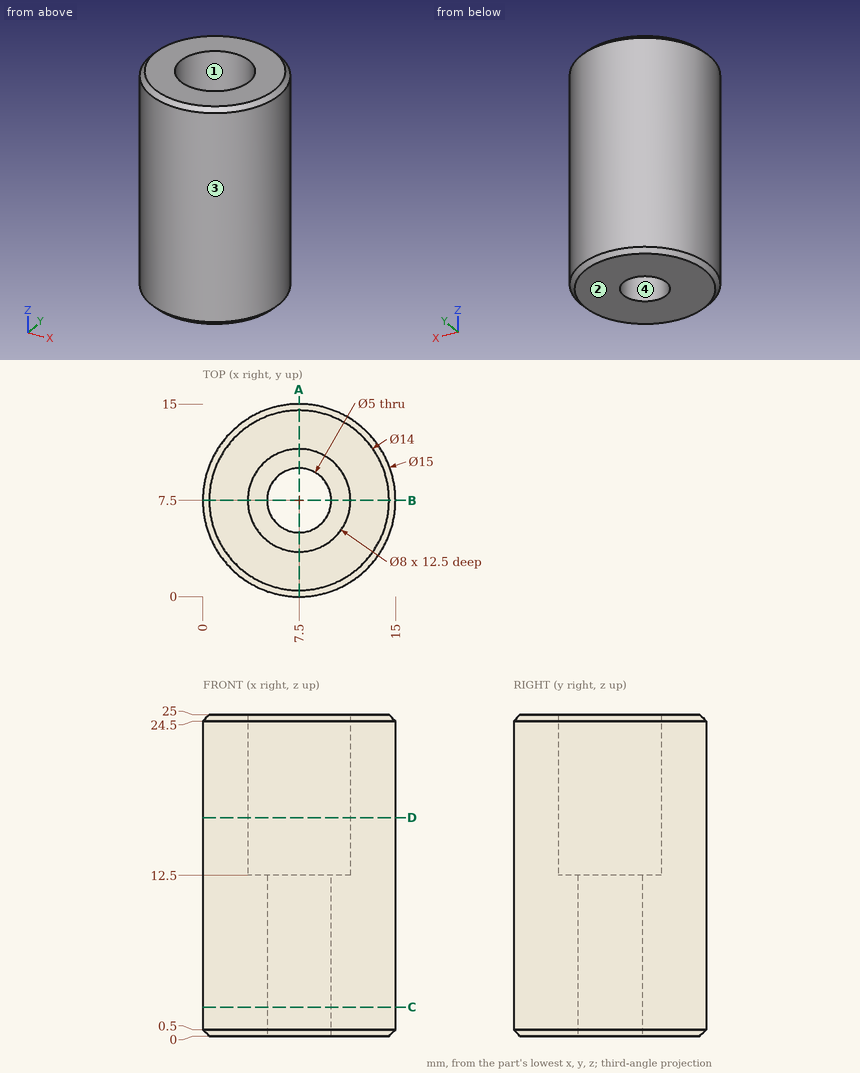
Geometry check sheet. Reference: drawing and pictorial views, mm from the part's lowest x, y, z. Round coordinates to 2 decimals unless told otherwise and drop trailing zeros. Loops run counter-clockwise (first coordinate to the right, second up) from the corner with the lowest first, then second, coordinate; pieces in that order, holes last. Notation, with made-up numbers: M 33.25,32 L 55.25,32 A34 ccw 55.25,69 Z; hole C 2.25,20 d7. An arc over 180 degrees is marked long. One line per item, written item: value.
(1) Sectioned sample at C-C, the plane z = 2.25. Record the cut outline in (x, y).
Computed values:
outline: C 7.5,7.5 d15; hole C 7.5,7.5 d5
(2) Depth check by flat-ended pin: pin 1 Ø8 at (x, y) = (5.5, 4.5) entering from -Z; pin 2 Ø5 at (y, z) = (11, 18.5) entering from +X; pin 3 Ø1.5 at (y, z) = (2, 14) entering from +X. Enter the tip coordinate at first touch or a pass-through.
Computed values:
pin 1: stops at z = 0
pin 2: stops at x = 14.93
pin 3: stops at x = 13.3
(3) Sectioned sample at D-D, the plane z = 17. Record the cut outline in (x, y), then the cut area to 3 significant figures.
Computed values:
outline: C 7.5,7.5 d15; hole C 7.5,7.5 d8
area: 126 mm^2
(4) Thickness scan on line 1 (Y direction, x = 7.5, z = 15.75); line 2 (Y direction, x = 7.5, z = 8.25); line 3 (Z direction, x = 6.5, y = 4). Record the ranges inside material, lowest first.
Computed values:
line 1: y = 0 to 3.5, 11.5 to 15
line 2: y = 0 to 5, 10 to 15
line 3: z = 0 to 12.5
(5) Release check for a two-part mould opening along X. For the marked faces 1, 2, 3 and 4 record: +X half, -X half, draft (parallel to the pull), parting line (faces both ways), or undercut.
Computed values:
face 1: undercut
face 2: draft
face 3: parting line
face 4: undercut
(6) Sectioned sample at A-A, the plane x = 7.5. Record the cut outline in (y, z).
Computed values:
outline: M 0,0.5 L 0.5,0 L 5,0 L 5,12.5 L 3.5,12.5 L 3.5,25 L 0.5,25 L 0,24.5 Z; M 10,0 L 14.5,0 L 15,0.5 L 15,24.5 L 14.5,25 L 11.5,25 L 11.5,12.5 L 10,12.5 Z
